Design review of the part shown in the three views and the two pictorial views. Dimensions are in mm from the part's minimum x, y and z. Round coordinates to 2 decimals unless told otherwise and drop trailing zeros. Loops run counter-clockwise (first coordinate to the right, second up) from the corner with the lowest first, then second, coordinate; pieces in that order, holes last. Notation, with made-up numbers: (-21, 78) -> (1, 78) arc R21 ccw to (1, 83) -> close; hole circle Ø7 at (8.25, -22.75). An arc over 180 degrees is marked (long way). Use a Markdown table: item, result. Add a question column.
1) Insertion check: pin 1 (1.5 mm diameter, centred on y = 9.5, z = 151, fed in from +X); pin 2 (10 mm diameter, centred on y = 8, z = 120, fed in from +X); pin 3 (4 mm diameter, centred on y = 5, z = 127, fed in from +X); pin 4 (11.5 mm diameter, centred on x = 13.5, y = 13.5, fed in from +Z). Each pin has a flat end and moves straight along its axis. Give the tip position at first contact, or say it passes through.
2) Consider section A-A on x = 13.5. Give the boundary of the cut face in (y, z) (1 decimal).
3) Consider section B-B on y = 19.5. Give the boundary of the cut face in (x, z), plus the area to 3 significant figures.
4) Wall thickness on probe 1 along X at (y, z) = (13.75, 65.5); probe 2 along Y at (x, z) = (13.5, 171.5) (1 decimal); probe 3 along Y at (x, z) = (18.25, 218) (1 decimal): over which ranges is each line inside the solid? List them lowest first.
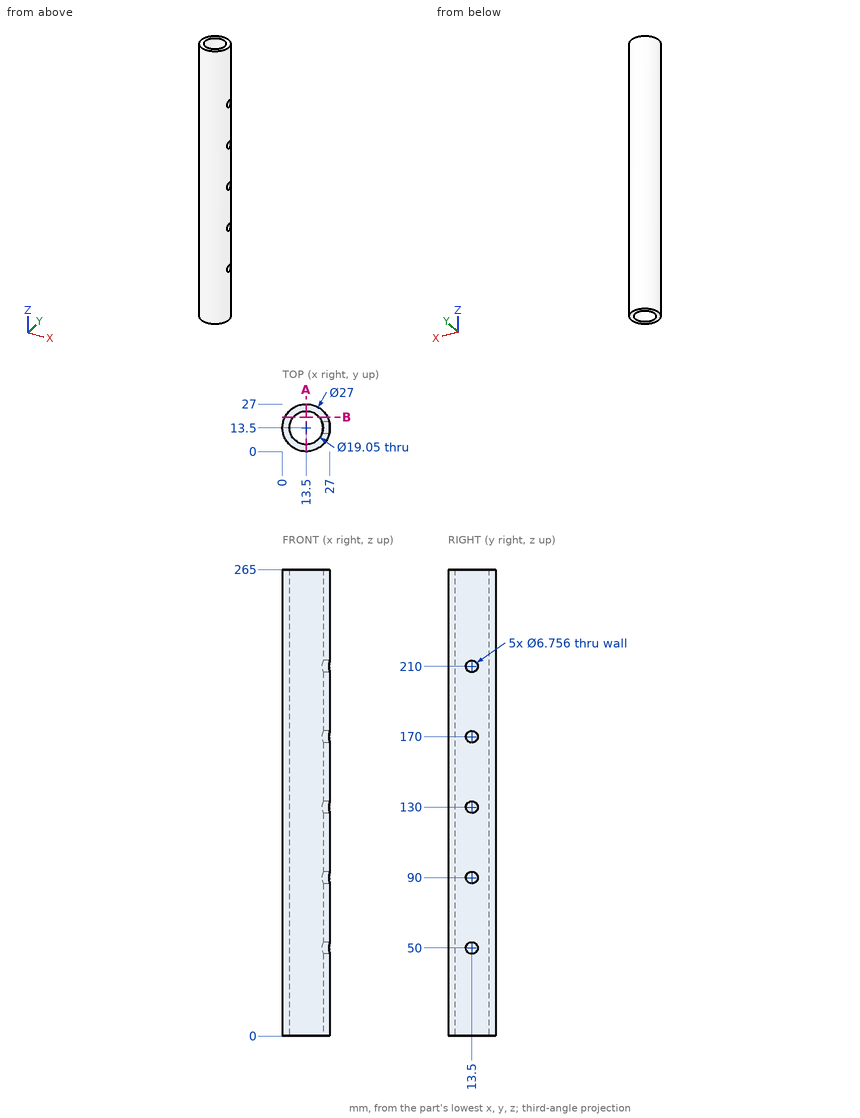
Result set:
| question | item | result |
|---|---|---|
| 1 | pin 1 | x = 26.6 |
| 1 | pin 2 | x = 26.99 |
| 1 | pin 3 | x = 25.33 |
| 1 | pin 4 | through |
| 2 | outline | (0, 0) -> (4, 0) -> (4, 265) -> (0, 265) -> close; (23, 0) -> (27, 0) -> (27, 265) -> (23, 265) -> close |
| 3 | outline | (1.41, 0) -> (6.1, 0) -> (6.1, 265) -> (1.41, 265) -> close; (20.9, 0) -> (25.59, 0) -> (25.59, 265) -> (20.9, 265) -> close |
| 3 | area | 2,490 mm2 |
| 4 | probe 1 | 0 to 3.98, 23.02 to 27 |
| 4 | probe 2 | 0 to 4, 23 to 27 |
| 4 | probe 3 | 0.9 to 5.2, 21.8 to 26.1 |
